```python
from build123d import *

# Parameters (mm, degrees)
CROQUIS1_R              = 3
SALIENTE_EXTRUIR1_DEPTH = 18
CROQUIS2_R              = 3
SALIENTE_EXTRUIR2_DEPTH = 18
SALIENTE_EXTRUIR3_DEPTH = 15
CROQUIS4_W              = 3
CROQUIS4_H              = 30
SALIENTE_EXTRUIR4_DEPTH = 95
CORTAR_EXTRUIR1_DEPTH   = 95


with BuildPart() as part:
    # Croquis1 → Saliente-Extruir1 (new body)
    with BuildSketch(Plane.XY):
        Circle(CROQUIS1_R)
    extrude(amount=SALIENTE_EXTRUIR1_DEPTH)

    # Croquis2 → Saliente-Extruir2 (add)
    with BuildSketch(Plane.XY):
        Circle(CROQUIS2_R)
    extrude(amount=-SALIENTE_EXTRUIR2_DEPTH)

    # Croquis3 → Saliente-Extruir3 (add)
    with BuildSketch(Plane(origin=(0, 0, 0), x_dir=(0, 0, -1), z_dir=(1, 0, 0))):
        Polygon((-18, -15), (-18, 0), (-18, 15), (-15, 15), (-15, -15), align=None)
        Polygon((18, 0), (18, 15), (15, 15), (15, -15), (18, -15), align=None)
    extrude(amount=SALIENTE_EXTRUIR3_DEPTH)

    # Croquis4 → Saliente-Extruir4 (add)
    with BuildSketch(Plane(origin=(0, 0, 0), x_dir=(0, 0, -1), z_dir=(1, 0, 0))):
        with Locations((16.5, 0)):
            Rectangle(CROQUIS4_W, CROQUIS4_H)
        with Locations((-16.5, 0)):
            Rectangle(CROQUIS4_W, CROQUIS4_H)
    extrude(amount=-SALIENTE_EXTRUIR4_DEPTH)

    # Croquis5 → Cortar-Extruir1 (cut)
    with BuildSketch(Plane.XY.offset(18)):
        with BuildLine():
            ThreePointArc((-95, 0), (-92.803300859, 5.303300859), (-87.5, 7.5))
            Line((-87.5, 7.5), (-2.55267423, 14.781199352))
            ThreePointArc((-2.55267423, 14.781199352), (-1.28101712, 14.945199736), (0, 15))
            Line((0, 15), (-95, 15))
            Line((-95, 15), (-95, 0))
        make_face()
        with BuildLine():
            ThreePointArc((-87.5, -7.5), (-92.803300859, -5.303300859), (-95, 0))
            Line((-95, 0), (-95, -15))
            Line((-95, -15), (0, -15))
            ThreePointArc((0, -15), (-1.28101712, -14.945199736), (-2.55267423, -14.781199352))
            Line((-2.55267423, -14.781199352), (-87.5, -7.5))
        make_face()
        with BuildLine():
            Line((15, -15), (15, 0))
            ThreePointArc((15, 0), (10.606601718, -10.606601718), (0, -15))
            Line((0, -15), (15, -15))
        make_face()
        with BuildLine():
            Line((15, 15), (0, 15))
            ThreePointArc((0, 15), (10.606601718, 10.606601718), (15, 0))
            Line((15, 0), (15, 15))
        make_face()
    extrude(amount=-CORTAR_EXTRUIR1_DEPTH, mode=Mode.SUBTRACT)


solid = part.part
```
Can you work these out from the model? Positions are in its coordinate system, mm. Coordinates: 2 decimals unless noted, no trailing zeros. Loops run counter-clockwise (first coordinate to the right, second up) from the corner with the lowest first, then second, coordinate; pieces in that order, holes last.
1) Thinking about a two-plate mould opening in Z: for faces 1 (the cylindrical face through (-3, 0, 0)), 2 (the flat face through (-41, 0, 15)), 3 (the flat face through (-39, 0, -18)), 4 (the flat face through (-44.43, -11.19, -16.48)), which applies, pulls with the +Z half, pulls with the -Z half, needs draft (parallel to the pull), parting line crosses it, or undercut?
2) Imagine slicing it at A-A on x = -54. List the corners of the cut face in (y, z) for me.
3) For pin 1 (5 mm diameter, centred on y = 3.5, z = 7.5, fed in from +X), with a flat end and sliding along its axis, tell me the tip position at first contact or that it passes through.
4) I need wall thicknesses on probe 1 along Z at (x, y) = (-1, -4); probe 2 along Y at (x, z) = (-37, 15.5); probe 3 along X at (y, z) = (-1.25, 6). Which ranges of each line are inside material? Lowest first, please.
5) Imagine slicing it at C-C on z = 1.5. List the corners of the cut face in (x, y) for me.
6) Imagine slicing it at B-B on y = -9.25. List the corners of the cut face in (x, z) for me, plus the area to 3 significant figures.
Completed:
1. face 1: undercut
1. face 2: undercut
1. face 3: pulls with the -Z half
1. face 4: needs draft
2. outline: (-10.37, -18) - (10.37, -18) - (10.37, -15) - (-10.37, -15) - close; (-10.37, 15) - (10.37, 15) - (10.37, 18) - (-10.37, 18) - close
3. pin 1: stops at x = 2.83
4. probe 1: z = -18 to -15, 15 to 18
4. probe 2: y = -11.83 to 11.83
4. probe 3: x = -2.73 to 2.73
5. outline: circle Ø6 at (0, 0)
6. outline: (-67.08, -18) - (11.81, -18) - (11.81, -15) - (-67.08, -15) - close; (-67.08, 15) - (11.81, 15) - (11.81, 18) - (-67.08, 18) - close
6. area: 473 mm2
